Part print with two shaded views. Sizes in mm from the minimum x, y, z corner. Coordinates: 2 decimals unless noted, no trailing zeros. Loops run counter-clockwise (first coordinate to the right, second up) from the corner with the lowest first, then second, coordinate; pieces in that order, holes last.
Item 1: Flat gauge pin, fed straight in: pin 1 (2.5 mm diameter, centred on x = 40.5, y = 19.5, fed in from -Z). Where does the tip first touch, or does it go through?
Item 2: Drill centre lines: line 1 along Y through (x, z) = (22.5, 0.75); line 2 along Y through (x, z) = (40.5, 2.25); line 3 along Y through (x, z) = (27.5, 2.05). Where is each one in solid material? Low to high.
Item 3: Cut at D-D (y = 11.25). List the corners of the cut face in (x, z).
Item 4: Cut at A-A (x = 22.5). List the corners of the cut face in (y, z), and give its area (3 significant figures).
Item 5: Cut at C-C (z = 1.95). Count the separate pieces of the cut face and the enclosed holes in it, and give its area (3 significant figures).
Item 6: Cut at B-B (x = 4.5). List the corners of the cut face in (y, z), and give its area (3 significant figures).
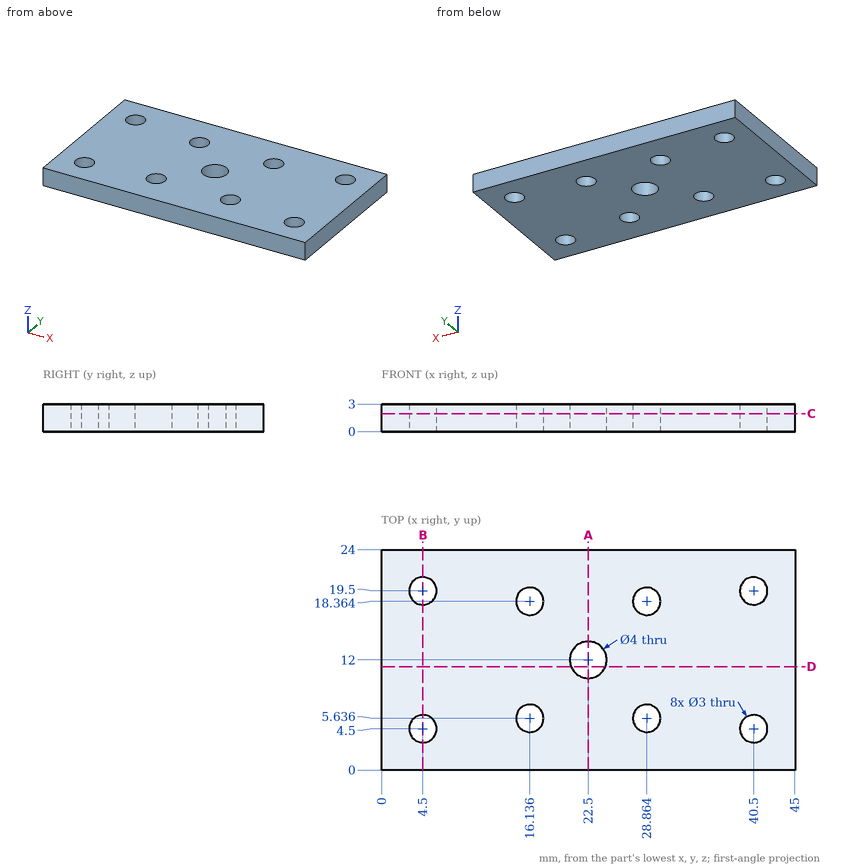
Filled sheet:
1. pin 1: passes through
2. line 1: y = 0 to 10, 14 to 24
2. line 2: y = 0 to 3, 6 to 18, 21 to 24
2. line 3: y = 0 to 5.01, 6.26 to 17.74, 18.99 to 24
3. outline: (0, 0) - (20.65, 0) - (20.65, 3) - (0, 3) - close; (24.35, 0) - (45, 0) - (45, 3) - (24.35, 3) - close
4. outline: (0, 0) - (10, 0) - (10, 3) - (0, 3) - close; (14, 0) - (24, 0) - (24, 3) - (14, 3) - close
4. area: 60.0 mm2
5. separate pieces: 1
5. enclosed holes: 9
5. area: 1,010 mm2
6. outline: (0, 0) - (3, 0) - (3, 3) - (0, 3) - close; (6, 0) - (18, 0) - (18, 3) - (6, 3) - close; (21, 0) - (24, 0) - (24, 3) - (21, 3) - close
6. area: 54.0 mm2
